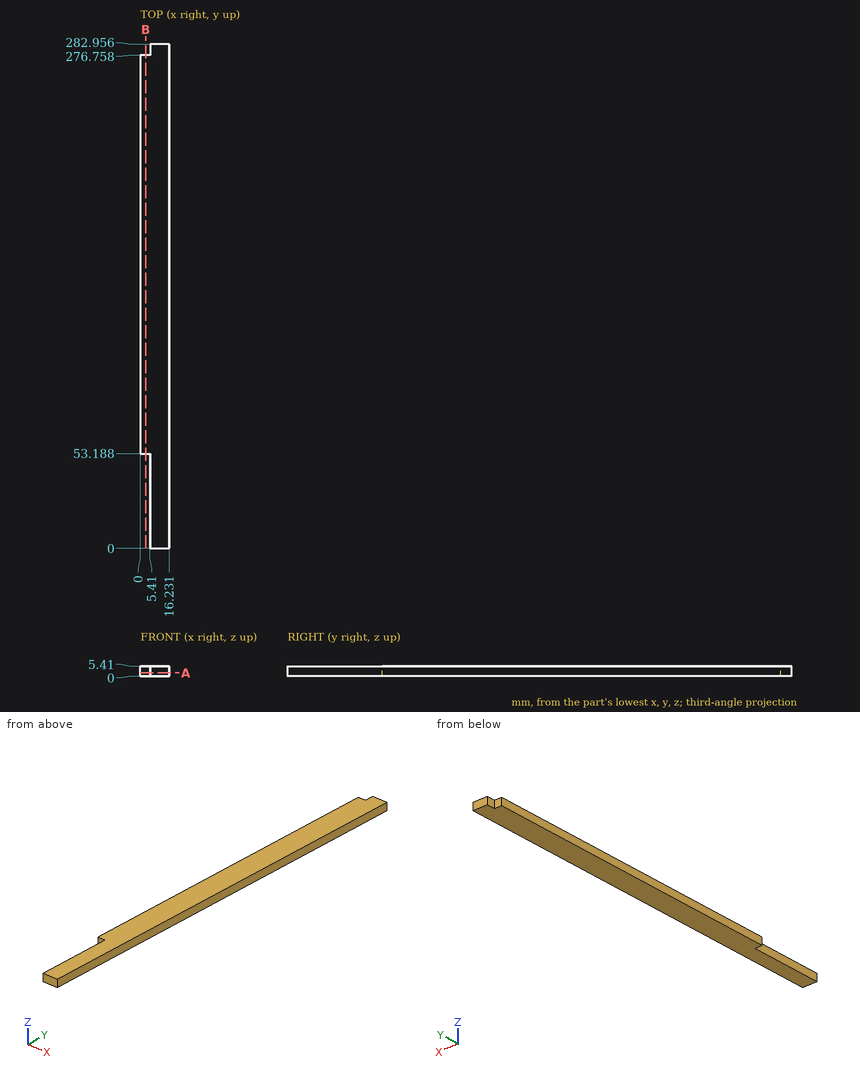
Geometry check sheet. Reference: drawing and pictorial views, mm from the part's lowest x, y, z. Round coordinates to 2 decimals unless told otherwise and drop trailing zeros. Order: outer loops, then holes, each group sorted by start corner. A loop starts at its lowest first (then second) coordinate and runs counter-clockwise, first axis right, second up.
Q1. Depth check by flat-ended pin: P1, Ø1.6, axis at y = 33, z = 2.5, coming from the -X side; P2, Ø1, axis at x = 7.5, z = 1.5, coming from the -Y side; P3, Ø2, axis at x = 3, z = 3, coming from the +Y side; P4, Ø1.6, axis at x = 2.5, z = 1.5, coming from the -Y side. Enter the tip coordinate at first touch or a pass-through.
Filled sheet:
P1: stops at x = 5.41
P2: stops at y = 0
P3: stops at y = 276.76
P4: stops at y = 53.19
Q2. Cross-section at A-A, the plane z = 1.7. Enter the section's corners in (x, y).
Filled sheet:
outline: (0, 53.19) - (5.41, 53.19) - (5.41, 0) - (16.23, 0) - (16.23, 282.96) - (5.41, 282.96) - (5.41, 276.76) - (0, 276.76) - close
Q3. Scan lines: L1, parallel to X at y = 22, z = 2.2; L2, parallel to Y at x = 5.25, z = 3.5. Record each from-to range of solid material in increasing order.
Filled sheet:
L1: x = 5.41 to 16.23
L2: y = 53.19 to 276.76
Q4. Cross-section at B-B, the plane x = 3. Enter the section's corners in (y, z), plus the area to 3 significant figures.
Filled sheet:
outline: (53.19, 0) - (276.76, 0) - (276.76, 5.41) - (53.19, 5.41) - close
area: 1,210 mm2
